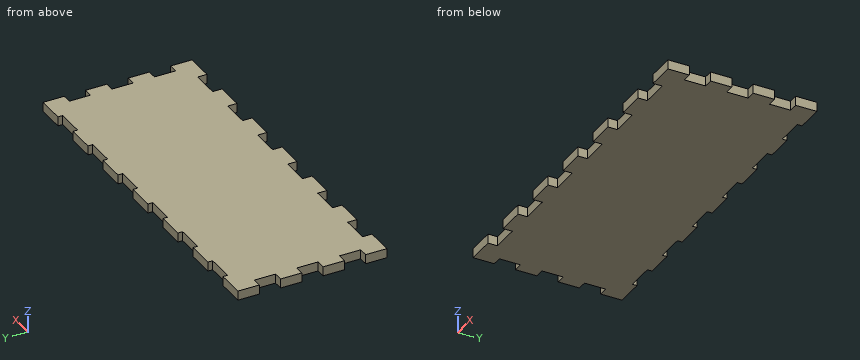
from build123d import *

# Parameters (mm, degrees)
ESBO_O1_W                = 231.5
ESBO_O1_H                = 96
RESSALTO_EXTRUS_O1_DEPTH = 6
CORTE_EXTRUS_O1_REACH    = 127.451
ESBO_O2_W                = 17.812307692
ESBO_O2_H                = 6
CORTE_EXTRUS_O3_REACH    = 127.451
ESBO_O4_W                = 6
ESBO_O4_H                = 13.715714286


with BuildPart() as part:
    # Esboço1 → Ressalto-extrusão1 (new body)
    with BuildSketch(Plane.XY):
        Rectangle(ESBO_O1_W, ESBO_O1_H)
    extrude(amount=RESSALTO_EXTRUS_O1_DEPTH)

    # Esboço2 → Corte-extrusão1 (cut, up to next)
    with BuildSketch(Plane(origin=(0, 0, 0), x_dir=(-1, 0, 0), z_dir=(0, 0, -1)), mode=Mode.PRIVATE) as corte_extrus_o1_sk1:
        with Locations((17.796153846, -45)):
            Rectangle(ESBO_O2_W, ESBO_O2_H)
    corte_extrus_o1_tool1 = extrude(corte_extrus_o1_sk1.sketch, amount=-CORTE_EXTRUS_O1_REACH, mode=Mode.PRIVATE) & part.part
    # Esboço2 → Corte-extrusão1 (cut, up to next)
    with BuildSketch(Plane(origin=(0, 0, 0), x_dir=(-1, 0, 0), z_dir=(0, 0, -1)), mode=Mode.PRIVATE) as corte_extrus_o1_sk2:
        with Locations((53.416153846, -45)):
            Rectangle(ESBO_O2_W, ESBO_O2_H)
    corte_extrus_o1_tool2 = extrude(corte_extrus_o1_sk2.sketch, amount=-CORTE_EXTRUS_O1_REACH, mode=Mode.PRIVATE) & part.part
    # Esboço2 → Corte-extrusão1 (cut, up to next)
    with BuildSketch(Plane(origin=(0, 0, 0), x_dir=(-1, 0, 0), z_dir=(0, 0, -1)), mode=Mode.PRIVATE) as corte_extrus_o1_sk3:
        with Locations((89.036153846, -45)):
            Rectangle(ESBO_O2_W, ESBO_O2_H)
    corte_extrus_o1_tool3 = extrude(corte_extrus_o1_sk3.sketch, amount=-CORTE_EXTRUS_O1_REACH, mode=Mode.PRIVATE) & part.part
    # Esboço2 → Corte-extrusão1 (cut, up to next)
    with BuildSketch(Plane(origin=(0, 0, 0), x_dir=(-1, 0, 0), z_dir=(0, 0, -1)), mode=Mode.PRIVATE) as corte_extrus_o1_sk4:
        with Locations((-17.823846154, -45)):
            Rectangle(ESBO_O2_W, ESBO_O2_H)
    corte_extrus_o1_tool4 = extrude(corte_extrus_o1_sk4.sketch, amount=-CORTE_EXTRUS_O1_REACH, mode=Mode.PRIVATE) & part.part
    # Esboço2 → Corte-extrusão1 (cut, up to next)
    with BuildSketch(Plane(origin=(0, 0, 0), x_dir=(-1, 0, 0), z_dir=(0, 0, -1)), mode=Mode.PRIVATE) as corte_extrus_o1_sk5:
        with Locations((-53.443846154, -45)):
            Rectangle(ESBO_O2_W, ESBO_O2_H)
    corte_extrus_o1_tool5 = extrude(corte_extrus_o1_sk5.sketch, amount=-CORTE_EXTRUS_O1_REACH, mode=Mode.PRIVATE) & part.part
    # Esboço2 → Corte-extrusão1 (cut, up to next)
    with BuildSketch(Plane(origin=(0, 0, 0), x_dir=(-1, 0, 0), z_dir=(0, 0, -1)), mode=Mode.PRIVATE) as corte_extrus_o1_sk6:
        with Locations((-89.063846154, -45)):
            Rectangle(ESBO_O2_W, ESBO_O2_H)
    corte_extrus_o1_tool6 = extrude(corte_extrus_o1_sk6.sketch, amount=-CORTE_EXTRUS_O1_REACH, mode=Mode.PRIVATE) & part.part
    # Esboço2 → Corte-extrusão1 (cut, up to next)
    with BuildSketch(Plane(origin=(0, 0, 0), x_dir=(-1, 0, 0), z_dir=(0, 0, -1)), mode=Mode.PRIVATE) as corte_extrus_o1_sk7:
        with Locations((-89.063846154, 48)):
            Rectangle(ESBO_O2_W, ESBO_O2_H)
    corte_extrus_o1_tool7 = extrude(corte_extrus_o1_sk7.sketch, amount=-CORTE_EXTRUS_O1_REACH, mode=Mode.PRIVATE) & part.part
    # Esboço2 → Corte-extrusão1 (cut, up to next)
    with BuildSketch(Plane(origin=(0, 0, 0), x_dir=(-1, 0, 0), z_dir=(0, 0, -1)), mode=Mode.PRIVATE) as corte_extrus_o1_sk8:
        with Locations((-53.443846154, 48)):
            Rectangle(ESBO_O2_W, ESBO_O2_H)
    corte_extrus_o1_tool8 = extrude(corte_extrus_o1_sk8.sketch, amount=-CORTE_EXTRUS_O1_REACH, mode=Mode.PRIVATE) & part.part
    # Esboço2 → Corte-extrusão1 (cut, up to next)
    with BuildSketch(Plane(origin=(0, 0, 0), x_dir=(-1, 0, 0), z_dir=(0, 0, -1)), mode=Mode.PRIVATE) as corte_extrus_o1_sk9:
        with Locations((-17.823846154, 48)):
            Rectangle(ESBO_O2_W, ESBO_O2_H)
    corte_extrus_o1_tool9 = extrude(corte_extrus_o1_sk9.sketch, amount=-CORTE_EXTRUS_O1_REACH, mode=Mode.PRIVATE) & part.part
    # Esboço2 → Corte-extrusão1 (cut, up to next)
    with BuildSketch(Plane(origin=(0, 0, 0), x_dir=(-1, 0, 0), z_dir=(0, 0, -1)), mode=Mode.PRIVATE) as corte_extrus_o1_sk10:
        with Locations((17.796153846, 48)):
            Rectangle(ESBO_O2_W, ESBO_O2_H)
    corte_extrus_o1_tool10 = extrude(corte_extrus_o1_sk10.sketch, amount=-CORTE_EXTRUS_O1_REACH, mode=Mode.PRIVATE) & part.part
    # Esboço2 → Corte-extrusão1 (cut, up to next)
    with BuildSketch(Plane(origin=(0, 0, 0), x_dir=(-1, 0, 0), z_dir=(0, 0, -1)), mode=Mode.PRIVATE) as corte_extrus_o1_sk11:
        with Locations((89.036153846, 48)):
            Rectangle(ESBO_O2_W, ESBO_O2_H)
    corte_extrus_o1_tool11 = extrude(corte_extrus_o1_sk11.sketch, amount=-CORTE_EXTRUS_O1_REACH, mode=Mode.PRIVATE) & part.part
    # Esboço2 → Corte-extrusão1 (cut, up to next)
    with BuildSketch(Plane(origin=(0, 0, 0), x_dir=(-1, 0, 0), z_dir=(0, 0, -1)), mode=Mode.PRIVATE) as corte_extrus_o1_sk12:
        with Locations((53.416153846, 48)):
            Rectangle(ESBO_O2_W, ESBO_O2_H)
    corte_extrus_o1_tool12 = extrude(corte_extrus_o1_sk12.sketch, amount=-CORTE_EXTRUS_O1_REACH, mode=Mode.PRIVATE) & part.part
    add(corte_extrus_o1_tool1.solids().sort_by_distance((-17.796154, -45, 0))[0], mode=Mode.SUBTRACT)
    add(corte_extrus_o1_tool2.solids().sort_by_distance((-53.416154, -45, 0))[0], mode=Mode.SUBTRACT)
    add(corte_extrus_o1_tool3.solids().sort_by_distance((-89.036154, -45, 0))[0], mode=Mode.SUBTRACT)
    add(corte_extrus_o1_tool4.solids().sort_by_distance((17.823846, -45, 0))[0], mode=Mode.SUBTRACT)
    add(corte_extrus_o1_tool5.solids().sort_by_distance((53.443846, -45, 0))[0], mode=Mode.SUBTRACT)
    add(corte_extrus_o1_tool6.solids().sort_by_distance((89.063846, -45, 0))[0], mode=Mode.SUBTRACT)
    add(corte_extrus_o1_tool7.solids().sort_by_distance((89.063846, 48, 0))[0], mode=Mode.SUBTRACT)
    add(corte_extrus_o1_tool8.solids().sort_by_distance((53.443846, 48, 0))[0], mode=Mode.SUBTRACT)
    add(corte_extrus_o1_tool9.solids().sort_by_distance((17.823846, 48, 0))[0], mode=Mode.SUBTRACT)
    add(corte_extrus_o1_tool10.solids().sort_by_distance((-17.796154, 48, 0))[0], mode=Mode.SUBTRACT)
    add(corte_extrus_o1_tool11.solids().sort_by_distance((-89.036154, 48, 0))[0], mode=Mode.SUBTRACT)
    add(corte_extrus_o1_tool12.solids().sort_by_distance((-53.416154, 48, 0))[0], mode=Mode.SUBTRACT)

    # Esboço4 → Corte-extrusão3 (cut, up to next)
    with BuildSketch(Plane(origin=(0, 0, 0), x_dir=(-1, 0, 0), z_dir=(0, 0, -1)), mode=Mode.PRIVATE) as corte_extrus_o3_sk1:
        with Locations((112.75, -0.002142857)):
            Rectangle(ESBO_O4_W, ESBO_O4_H)
    corte_extrus_o3_tool1 = extrude(corte_extrus_o3_sk1.sketch, amount=-CORTE_EXTRUS_O3_REACH, mode=Mode.PRIVATE) & part.part
    # Esboço4 → Corte-extrusão3 (cut, up to next)
    with BuildSketch(Plane(origin=(0, 0, 0), x_dir=(-1, 0, 0), z_dir=(0, 0, -1)), mode=Mode.PRIVATE) as corte_extrus_o3_sk2:
        with Locations((112.75, 27.427857143)):
            Rectangle(ESBO_O4_W, ESBO_O4_H)
    corte_extrus_o3_tool2 = extrude(corte_extrus_o3_sk2.sketch, amount=-CORTE_EXTRUS_O3_REACH, mode=Mode.PRIVATE) & part.part
    # Esboço4 → Corte-extrusão3 (cut, up to next)
    with BuildSketch(Plane(origin=(0, 0, 0), x_dir=(-1, 0, 0), z_dir=(0, 0, -1)), mode=Mode.PRIVATE) as corte_extrus_o3_sk3:
        with Locations((-112.75, 27.427857143)):
            Rectangle(ESBO_O4_W, ESBO_O4_H)
    corte_extrus_o3_tool3 = extrude(corte_extrus_o3_sk3.sketch, amount=-CORTE_EXTRUS_O3_REACH, mode=Mode.PRIVATE) & part.part
    # Esboço4 → Corte-extrusão3 (cut, up to next)
    with BuildSketch(Plane(origin=(0, 0, 0), x_dir=(-1, 0, 0), z_dir=(0, 0, -1)), mode=Mode.PRIVATE) as corte_extrus_o3_sk4:
        with Locations((-112.75, -0.002142857)):
            Rectangle(ESBO_O4_W, ESBO_O4_H)
    corte_extrus_o3_tool4 = extrude(corte_extrus_o3_sk4.sketch, amount=-CORTE_EXTRUS_O3_REACH, mode=Mode.PRIVATE) & part.part
    # Esboço4 → Corte-extrusão3 (cut, up to next)
    with BuildSketch(Plane(origin=(0, 0, 0), x_dir=(-1, 0, 0), z_dir=(0, 0, -1)), mode=Mode.PRIVATE) as corte_extrus_o3_sk5:
        with Locations((-112.75, -27.432142857)):
            Rectangle(ESBO_O4_W, ESBO_O4_H)
    corte_extrus_o3_tool5 = extrude(corte_extrus_o3_sk5.sketch, amount=-CORTE_EXTRUS_O3_REACH, mode=Mode.PRIVATE) & part.part
    # Esboço4 → Corte-extrusão3 (cut, up to next)
    with BuildSketch(Plane(origin=(0, 0, 0), x_dir=(-1, 0, 0), z_dir=(0, 0, -1)), mode=Mode.PRIVATE) as corte_extrus_o3_sk6:
        with Locations((112.75, -27.432142857)):
            Rectangle(ESBO_O4_W, ESBO_O4_H)
    corte_extrus_o3_tool6 = extrude(corte_extrus_o3_sk6.sketch, amount=-CORTE_EXTRUS_O3_REACH, mode=Mode.PRIVATE) & part.part
    add(corte_extrus_o3_tool1.solids().sort_by_distance((-112.75, -0.002143, 0))[0], mode=Mode.SUBTRACT)
    add(corte_extrus_o3_tool2.solids().sort_by_distance((-112.75, 27.427857, 0))[0], mode=Mode.SUBTRACT)
    add(corte_extrus_o3_tool3.solids().sort_by_distance((112.75, 27.427857, 0))[0], mode=Mode.SUBTRACT)
    add(corte_extrus_o3_tool4.solids().sort_by_distance((112.75, -0.002143, 0))[0], mode=Mode.SUBTRACT)
    add(corte_extrus_o3_tool5.solids().sort_by_distance((112.75, -27.432143, 0))[0], mode=Mode.SUBTRACT)
    add(corte_extrus_o3_tool6.solids().sort_by_distance((-112.75, -27.432143, 0))[0], mode=Mode.SUBTRACT)


solid = part.part
The listing builds one solid part. Answer for the finished solid, in the listing's coordinates (mm). Round coordinates to 2 decimals unless told otherwise and drop trailing zeros. Order: outer loops, then holes, each group sorted by start corner. A loop starts at its lowest first (then second) coordinate and runs counter-clockwise, first axis right, second up. Notation, with made-up numbers: (-26, 33.5) -> (15, 33.5) arc R33 cw to (15, 64.5) -> close; hole circle Ø7 at (3.5, -8.75). An arc over 180 degrees is marked (long way). Write each question's results on one line, items separated by ' | '. Start each with the question number.
Q1. Each of these flat-tipped pins is pushed along its axis until it touches: pin 1 (12 mm diameter, centred on x = -10, y = -30.5, fed in from -Z); pin 2 (3 mm diameter, centred on y = 28.5, z = 5, fed in from -X); pin 3 (3 mm diameter, centred on x = -89.5, z = 3, fed in from -Y). Where does it stop, or does it pass through?
Q2. Find section A-A (x = 21). Determine the outline of the cut face in (y, z).
Q3. Straight lines are drawn through the part: probe 1 along Y at (x, z) = (-21.5, 5.7); probe 2 along X at (y, z) = (-2, 1.05). For each, find the intervals that lie inside material, in ascending order. Write a range as from..to.
Q4. Find section B-B (y = -27.5). Determine the outline of the cut face in (x, z), then the cut area to 3 significant figures.
Worked answers:
1) pin 1: stops at z = 0 | pin 2: stops at x = -109.75 | pin 3: stops at y = -42
2) outline: (-42, 0) -> (45, 0) -> (45, 6) -> (-42, 6) -> close
3) probe 1: y = -42..45 | probe 2: x = -109.75..109.75
4) outline: (-109.75, 0) -> (109.75, 0) -> (109.75, 6) -> (-109.75, 6) -> close | area: 1,320 mm2
